```python
from build123d import *

# Parameters (mm, degrees)
F1_DEPTH  = 4
F2_W      = 22
F2_H      = 8.5
F2_W_2    = 37
F2_H_2    = 6
F3_DEPTH  = 14
F4_R      = 6.2
F5_DEPTH  = 8.5
F6_R      = 12.5
F7_DEPTH  = 32.001
F8_R      = 8.2
F9_DEPTH  = 2
F10_R     = 8.2
F11_DEPTH = 2
F12_R     = 1.5
F13_DEPTH = 18.001
F14_R     = 1.6
F15_DEPTH = 4
F16_R     = 1.6
F17_DEPTH = 18.001
F18_R     = 3.25
F19_DEPTH = 1.6
F20_R     = 3.25
F21_DEPTH = 15.6


with BuildPart() as f1:
    # F0 (on Top) → F1 (new body)
    with BuildSketch(Plane.XY):
        with BuildLine():
            Line((4, 0), (18.5, 0))
            Line((18.5, 0), (18.5, 30))
            Line((18.5, 30), (11, 30))
            Line((11, 30), (11, 45))
            Line((11, 45), (-11, 45))
            Line((-11, 45), (-11, 30))
            Line((-11, 30), (-18.5, 30))
            Line((-18.5, 30), (-18.5, 0))
            Line((-18.5, 0), (-4, 0))
            ThreePointArc((-4, 0), (0, -2), (4, 0))
        make_face()
        with BuildLine():
            Line((-12.5, 6), (-12.5, 24))
            Line((-12.5, 24), (12.5, 24))
            Line((12.5, 24), (12.5, 6))
            Line((12.5, 6), (4, 6))
            ThreePointArc((4, 6), (0, 8), (-4, 6))
            Line((-4, 6), (-12.5, 6))
        make_face(mode=Mode.SUBTRACT)
    extrude(amount=F1_DEPTH)

    # F2 (on face) → F3 (join)
    with BuildSketch(Plane.XY.offset(4)):
        with Locations((0, 40.75)):
            Rectangle(F2_W, F2_H)
        with Locations((0, 27)):
            Rectangle(F2_W_2, F2_H_2)
        with Locations((0, 3)):
            Rectangle(F2_W_2, F2_H_2)
    extrude(amount=F3_DEPTH)

    # F4 (on face) → F5 (cut, through all)
    with BuildSketch(Plane(origin=(0, 45, 0), x_dir=(-1, 0, 0), z_dir=(0, 1, 0))):
        with Locations((0, 18)):
            Circle(F4_R)
    extrude(amount=-F5_DEPTH, mode=Mode.SUBTRACT)

    # F6 (on face) → F7 (cut, through all)
    with BuildSketch(Plane(origin=(0, 30, 0), x_dir=(-1, 0, 0), z_dir=(0, 1, 0))):
        with Locations((0, 18)):
            Circle(F6_R)
    extrude(amount=-F7_DEPTH, mode=Mode.SUBTRACT)

    # F8 (on face) → F9 (cut)
    with BuildSketch(Plane(origin=(0, 45, 0), x_dir=(-1, 0, 0), z_dir=(0, 1, 0))):
        with Locations((0, 18)):
            Circle(F8_R)
    extrude(amount=-F9_DEPTH, mode=Mode.SUBTRACT)

    # F10 (on face) → F11 (cut)
    with BuildSketch(Plane.XZ.offset(-36.5)):
        with Locations((0, 18)):
            Circle(F10_R)
    extrude(amount=-F11_DEPTH, mode=Mode.SUBTRACT)

    # F12 (on face) → F13 (cut, through all)
    with BuildSketch(Plane(origin=(0, 0, 0), x_dir=(1, 0, 0), z_dir=(0, 0, -1))):
        with Locations((-15.5, -27)):
            Circle(F12_R)
        with Locations((15.5, -27)):
            Circle(F12_R)
        with Locations((15.5, -3)):
            Circle(F12_R)
        with Locations((-15.5, -3)):
            Circle(F12_R)
    extrude(amount=-F13_DEPTH, mode=Mode.SUBTRACT)

    # F14 (on face) → F15 (cut, through all)
    with BuildSketch(Plane.XY.offset(4)):
        with Locations((0, 33.25)):
            Circle(F14_R)
    extrude(amount=-F15_DEPTH, mode=Mode.SUBTRACT)

    # F16 (on face) → F17 (cut, through all)
    with BuildSketch(Plane(origin=(0, 0, 0), x_dir=(1, 0, 0), z_dir=(0, 0, -1))):
        with Locations((0, -3)):
            Circle(F16_R)
    extrude(amount=-F17_DEPTH, mode=Mode.SUBTRACT)

    # F18 (on face) → F19 (cut)
    with BuildSketch(Plane.XY.offset(4)):
        with Locations((0, 3)):
            Circle(F18_R)
        with Locations((0, 33.25)):
            Circle(F18_R)
    extrude(amount=-F19_DEPTH, mode=Mode.SUBTRACT)

    # F20 (on face) → F21 (cut, through all)
    with BuildSketch(Plane.XY.offset(2.4)):
        with Locations((0, 3)):
            Circle(F20_R)
    extrude(amount=F21_DEPTH, mode=Mode.SUBTRACT)


solid = f1.part
```
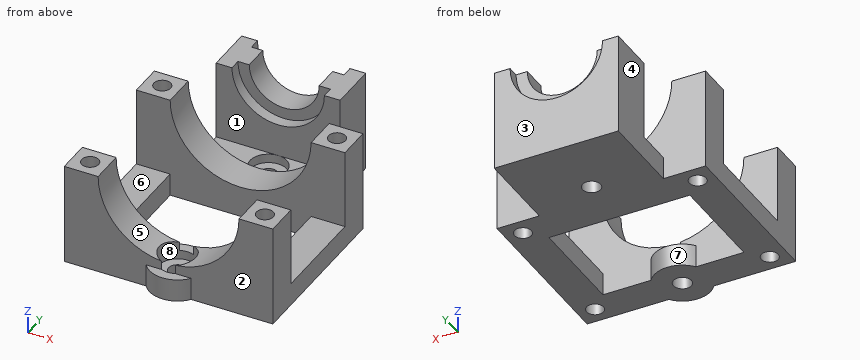
Geometry: final body of the model. Coordinates: model frame, mm. Face numbers are marked on the shaded views. A direction names the side the tool comes from. Coordinates: 2 decimals unless noted, no trailing zeros. Order: outer loops, then holes, each group sorted by start corner. A loop starts at its lowest first (then second) coordinate and runs counter-clockwise, first axis right, second up. Notation, with made-up numbers: (84.5, -32.75) - (97.5, -32.75) arc R16 cw to (97.5, -6.75) - close; hole circle Ø10 at (54, 36.25). An arc over 180 degrees is marked (long way). Return JSON: item names as keys, results as strings. Group by question number.
1. Pin query (flat end, axial travel): pin 1 (8 mm diameter, centred on x = -11.5, y = 14, fed in from +Z); pin 2 (2.5 mm diameter, centred on x = 15.5, y = 27, fed in from -Z); pin 3 (5 mm diameter, centred on x = -8.5, z = 14.5, fed in from -Y); pin 4 (6.5 mm diameter, centred on x = 1.5, z = 13.5, fed in from -Y). Return the tip coordinate at first contact, or that it passes through.
2. Cut plane A-A (y = 27). Output: boundary loops of the cut face in (x, z).
3. Set-up query: the marked faces 4, 5, 6, 7 and 8. Return all of +Z, -Z, +X, -X, +Y, -Y with unobstructed straight access to the full face (end or side cutting, diameter ignored); none if empty.
4. Cut plane C-C (x = 15.5). Output: boundary loops of the cut face in (y, z).
5. Cut plane D-D (y = 9). Output: boundary loops of the cut face in (x, z).
6. Material intervals for line 1 along Y through (x, z) = (-15.5, 8); line 2 along X through (y, z) = (3, 5.5); line 3 along X through (y, z) = (33.25, 3.3), sorted ascending. Write a range as [from, to].
7. Cut plane B-B (z = 6.75). Count the separate pieces of the cut face and the enclosed holes in it, plus the area to 3 significant figures.
8. Pull-direction query (Y, two-part tool) for the marked faces 1, 2 and 3; classes: pulls with the +Y half, pulls with the -Y half, needs draft (parallel to the pull), parting line crosses it, or undercut.
Resolved:
{
 "1": {"pin 1": "stops at z = 4", "pin 2": "passes through", "pin 3": "stops at y = 36.5", "pin 4": "stops at y = 38.5"},
 "2": {"outline": "(-18.5, 0) - (-17, 0) - (-17, 18) - (-18.5, 18) - close; (-14, 0) - (14, 0) - (14, 18) - (12.5, 18) arc R12.5 cw to (-12.5, 18) - (-14, 18) - close; (17, 0) - (18.5, 0) - (18.5, 18) - (17, 18) - close"},
 "3": {"face 4": "+Z, -Z, -X, +Y", "face 5": "+Z, -Y", "face 6": "+Z, +X, -X", "face 7": "+Z, -Z", "face 8": "+Z"},
 "4": {"outline": "(0, 0) - (1.5, 0) - (1.5, 18) - (0, 18) - close; (4.5, 0) - (25.5, 0) - (25.5, 18) - (24, 18) - (24, 4) - (6, 4) - (6, 18) - (4.5, 18) - close; (28.5, 0) - (30, 0) - (30, 18) - (28.5, 18) - close"},
 "5": {"outline": "(-18.5, 0) - (-12.5, 0) - (-12.5, 4) - (-18.5, 4) - close; (12.5, 0) - (18.5, 0) - (18.5, 4) - (12.5, 4) - close"},
 "6": {"line 1": "y = [0, 1.5], [4.5, 6], [24, 25.5], [28.5, 30]", "line 2": "x = [-18.5, -17], [-14, -3.25], [3.25, 14], [17, 18.5]", "line 3": "x = [-11, -3.25], [3.25, 11]"},
 "7": {"separate pieces": "5", "enclosed holes": "4", "area": "472 mm²"},
 "8": {"face 1": "undercut", "face 2": "pulls with the -Y half", "face 3": "pulls with the +Y half"}
}
